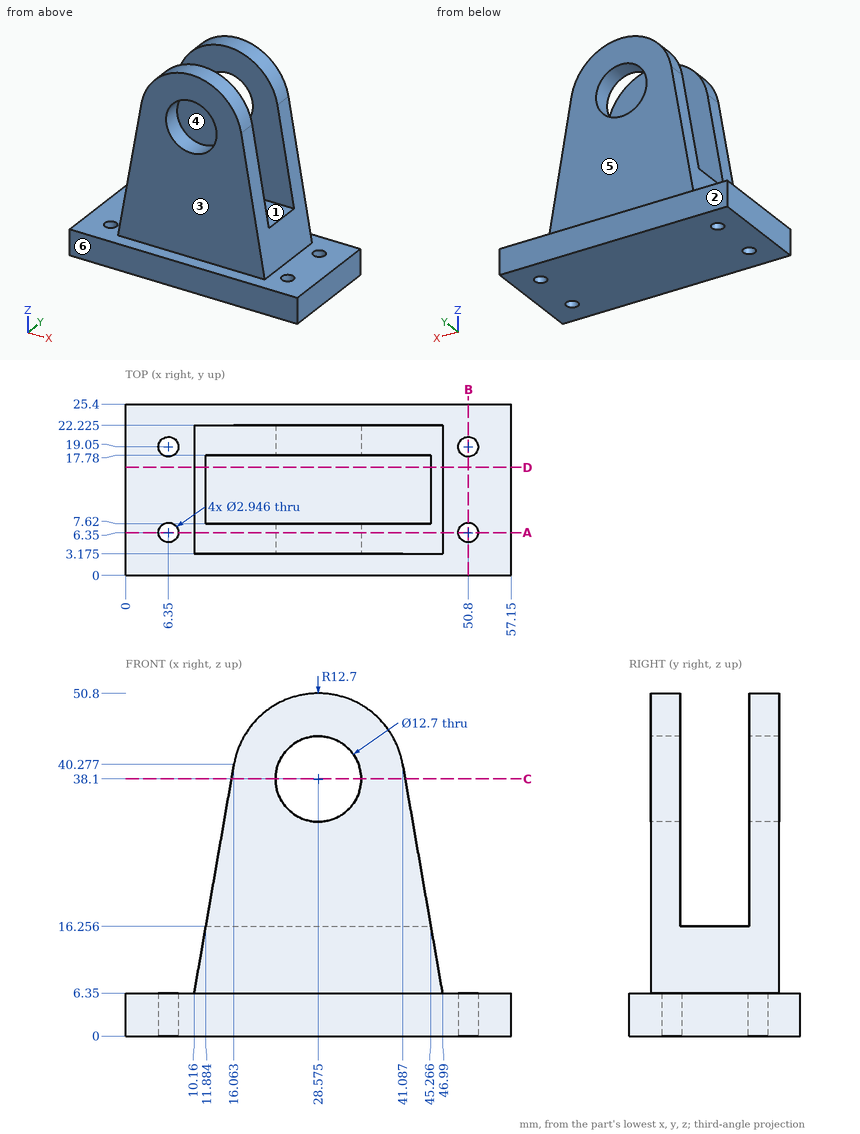
Can you work these out from the drawing? Everything is in mm from the part's minimum corner. A direction names the side the tool comes from. Coordinates: 2 decimals unless noted, no trailing zeros. Write each loop counter-clockwise with the first axis right and the second up, starting at its lowest first coordinate (ties: lowest second). Pieces come first, ordered by that corner, then holes. Notation, with made-up numbers: (-22.75, 7) -> (2.25, 7) arc R17 ccw to (2.25, 38) -> close; hole circle Ø5 at (18.5, 33.25). An arc over 180 degrees is marked (long way). Write each question's results on one line, items separated by ' | '. Start each with the question number.
Q1. Imagine slicing it at B-B (x = 50.8). Write out the boundary of the cut face in (y, z), then the cut area to 3 significant figures.
Q2. On a 3-axis mill with a long thin cutter (end or side, diameter ignored), from which of +Z, -Z, +X, -X, +Y, -Y can I reach the whole of each face in a straight line? I mean the marked faces 1, 2 and 3. Say none if no direction works.
Q3. If I drill on probe 1 along Y at (x, z) = (23, 46.5) (1 decimal); probe 2 along Y at (x, z) = (6, 2); probe 3 along Z at (x, y) = (52, 24.25), over which ranges is the centre line in solid material (lowest first)?
Q4. I'm going to push flat-ended pins straight in: pin 1 (12 mm diameter, centred on x = 14.5, y = 13.5, fed in from +Z); pin 2 (1 mm diameter, centred on x = 35.5, y = 4.5, fed in from -Z); pin 3 (11.5 mm diameter, centred on x = 28.575, z = 38.1, fed in from -Y); pin 4 (1 mm diameter, centred on y = 7.5, z = 37, fed in from -X). Where does each tip first touch, or does it pass through?
Q5. We'd pull the mould along Y, two halves only. Please class the marked faces 4, 5 and 6: +Y half, -Y half, draft (parallel to the pull), parting line (faces both ways), or undercut.
Q6. Imagine slicing it at C-C (z = 38.1). Write out the boundary of the cut face in (x, y) (1 decimal).
Q7. Imagine slicing it at D-D (y = 16). Write out the boundary of the cut face in (x, z).
Q8. Imagine slicing it at A-A (y = 6.35). State how many separate pieces and enclosed holes the cut face has, then the cut area to 3 significant figures.
Taken from the geometry:
1) outline: (0, 0) -> (4.88, 0) -> (4.88, 6.35) -> (0, 6.35) -> close; (7.82, 0) -> (17.58, 0) -> (17.58, 6.35) -> (7.82, 6.35) -> close; (20.52, 0) -> (25.4, 0) -> (25.4, 6.35) -> (20.52, 6.35) -> close | area: 124 mm^2
2) face 1: +Z, +X, -X | face 2: +Z, -Z, +X, -X, +Y | face 3: +Z, +X, -X, -Y
3) probe 1: y = 3.2 to 7.6, 17.8 to 22.2 | probe 2: y = 0 to 4.92, 7.78 to 17.62, 20.48 to 25.4 | probe 3: z = 0 to 6.35
4) pin 1: stops at z = 46.09 | pin 2: stops at z = 0 | pin 3: passes through | pin 4: stops at x = 15.41
5) face 4: undercut | face 5: +Y half | face 6: -Y half
6) outline: (15.7, 3.2) -> (22.2, 3.2) -> (22.2, 7.6) -> (15.7, 7.6) -> close; (15.7, 17.8) -> (22.2, 17.8) -> (22.2, 22.2) -> (15.7, 22.2) -> close; (34.9, 3.2) -> (41.5, 3.2) -> (41.5, 7.6) -> (34.9, 7.6) -> close; (34.9, 17.8) -> (41.5, 17.8) -> (41.5, 22.2) -> (34.9, 22.2) -> close
7) outline: (0, 0) -> (57.15, 0) -> (57.15, 6.35) -> (46.99, 6.35) -> (45.27, 16.26) -> (11.88, 16.26) -> (10.16, 6.35) -> (0, 6.35) -> close
8) separate pieces: 3 | enclosed holes: 1 | area: 1,450 mm^2
